```python
from build123d import *

# Parameters (mm, degrees)
BOSS_EXTRUDE1_DEPTH = 1.8
SKETCH2_R           = 2.500000000000001
BOSS_EXTRUDE2_DEPTH = 3
SKETCH3_R           = 2.5000000000000013
BOSS_EXTRUDE3_DEPTH = 0.5
CHAMFER1_SIZE       = 0.4
SKETCH4_W           = 0.5
SKETCH4_H           = 1.7000000000000002
BOSS_EXTRUDE4_DEPTH = 0.2
CHAMFER2_SIZE       = 0.3
CHAMFER2_SIZE_2     = 0.221880218
FILLET1_R           = 0.2


with BuildPart() as part:
    # Sketch1 → Boss-Extrude1 (new body)
    with BuildSketch(Plane(origin=(0, 0, 0), x_dir=(1, 0, 0), z_dir=(0, 1, 0))):
        with BuildLine():
            Line((-3, -6.5), (-3.0000000000000027, 6.499999999999998))
            ThreePointArc((-3.0000000000000027, 6.499999999999998), (-4.2e-15, 9.5), (2.9999999999999973, 6.500000000000002))
            Line((2.9999999999999973, 6.500000000000002), (3, -6.5))
            ThreePointArc((3, -6.5), (-5.5e-16, -9.5), (-3, -6.5))
        make_face()
    extrude(amount=BOSS_EXTRUDE1_DEPTH)

    # Sketch2 → Boss-Extrude2 (add)
    with BuildSketch(Plane(origin=(0, 1.8, 0), x_dir=(1, 0, 0), z_dir=(0, 1, 0))):
        with Locations(Location((-2.39e-15, 6.5, 0), (0, 0, 270))):
            Circle(SKETCH2_R)
        with Locations(Location((0, -6.5, 0), (0, 0, 270))):
            Circle(SKETCH2_R)
    extrude(amount=BOSS_EXTRUDE2_DEPTH)

    # Sketch3 → Boss-Extrude3 (add)
    with BuildSketch(Plane(origin=(0, 4.800000000000001, 0), x_dir=(1, 0, 0), z_dir=(0, 1, 0))):
        with Locations(Location((-2.39e-15, 6.5, 0), (0, 0, 270))):
            Circle(SKETCH3_R)
    extrude(amount=BOSS_EXTRUDE3_DEPTH)

    # Chamfer1
    chamfer1_edges = [part.edges().sort_by_distance(p)[0] for p in [
        (7.7e-16, 4.8, 3.999999999999999),
        (-1.62e-15, 5.300000000000001, -9.000000000000002),
    ]]
    chamfer(chamfer1_edges, length=CHAMFER1_SIZE)

    # Sketch4 → Boss-Extrude4 (add)
    with BuildSketch(Plane(origin=(0, 5.300000000000001, 0), x_dir=(1, 0, 0), z_dir=(0, 1, 0))):
        with BuildLine():
            Line((-0.75, 7.913329402510258), (-0.75, 7.304673846971556))
            ThreePointArc((-0.75, 7.304673846971556), (-4.54e-15, 5.4), (0.75, 7.304673846971556))
            Line((0.75, 7.304673846971556), (0.75, 7.913329402510258))
            ThreePointArc((0.75, 7.913329402510258), (-5.52e-15, 4.9), (-0.75, 7.913329402510258))
        make_face()
        with Locations((-2.76e-15, 7.449999999999999)):
            Rectangle(SKETCH4_W, SKETCH4_H)
    extrude(amount=BOSS_EXTRUDE4_DEPTH)

    # Chamfer2
    # the kernel refuses this chamfer: 0.3, 0.221880218 mm, written as the material it takes off along each edge
    with BuildSketch(Plane(origin=(-0.75, 5.300000000000001, -7.913329402510258), x_dir=(0, 0, 1), z_dir=(0, 1, 0))) as chamfer2_piece_1:
        with BuildLine():
            Line((CHAMFER2_SIZE, 0), (0.11497408326020686, -0.18502591673979885))
            ThreePointArc((0.11497408326020686, -0.18502591673979885), (0.05505412011014688, -0.09562891224277614), (0, 0))
            Line((0, 0), (CHAMFER2_SIZE, 0))
        make_face()
    extrude(amount=0.9715048963897726, mode=Mode.SUBTRACT)
    with BuildSketch(Plane(origin=(0.75, 5.300000000000001, -7.913329402510258), x_dir=(0.8394299671515956, 0, 0.5434678741635711), z_dir=(0, 1, 0))) as chamfer2_piece_2:
        with BuildLine():
            Line((0.27705330102285075, 2e-17), (CHAMFER2_SIZE_2 * 0.543467874804, -CHAMFER2_SIZE_2 * 0.83942996814))
            Line((CHAMFER2_SIZE_2 * 0.543467874804, -CHAMFER2_SIZE_2 * 0.83942996814), (0, 0))
            ThreePointArc((0, 0), (0.14238943823073183, 0.00600337759415658), (0.27705330102285075, 2e-17))
        make_face()
    extrude(amount=0.9123006442989672, mode=Mode.SUBTRACT)

    # Fillet1
    # the kernel refuses this fillet: 0.2 mm, written as the material it takes off along each edge
    with BuildSketch(Plane(origin=(-0.7500000000000032, 5.500000000000001, -6.599999999999999), x_dir=(0, -1, 0), z_dir=(1, 0, 0))) as fillet1_piece_1:
        with BuildLine():
            CenterArc((FILLET1_R, FILLET1_R), FILLET1_R, 180, 90)
            Line((0, FILLET1_R), (0, 0))
            Line((0, 0), (FILLET1_R, 0))
        make_face()
    extrude(amount=1.5000000000000009, mode=Mode.SUBTRACT)
    with BuildSketch(Plane(origin=(-0.2500000000000028, 5.500000000000001, -8.799999999999999), x_dir=(0, -1, 0), z_dir=(0, 0, 1)), Plane(origin=(0.24999999999999725, 5.500000000000001, -6.099999999999998), x_dir=(0, -1, 0), z_dir=(0, 0, -1))) as fillet1_piece_2:
        with BuildLine():
            CenterArc((FILLET1_R, FILLET1_R), FILLET1_R, 180, 90)
            Line((0, FILLET1_R), (0, 0))
            Line((0, 0), (FILLET1_R, 0))
        make_face()
    extrude(amount=2.700000000000001, mode=Mode.SUBTRACT)
    with BuildSketch(Plane(origin=(0.7499999999999977, 5.500000000000001, -8.299999999999999), x_dir=(0, -1, 0), z_dir=(-1, 0, 0))) as fillet1_piece_3:
        with BuildLine():
            CenterArc((FILLET1_R, FILLET1_R), FILLET1_R, 180, 90)
            Line((0, FILLET1_R), (0, 0))
            Line((0, 0), (FILLET1_R, 0))
        make_face()
    extrude(amount=1.5000000000000009, mode=Mode.SUBTRACT)
    with BuildSketch(Plane(origin=(-0.75, 5.500000000000001, -8.11332940251), x_dir=(0, -1, 0), z_dir=(0, 0, 1))) as fillet1_piece_4:
        with BuildLine():
            CenterArc((FILLET1_R, -FILLET1_R), FILLET1_R, 90, 90)
            Line((0, -FILLET1_R), (0, 0))
            Line((0, 0), (FILLET1_R, 0))
        make_face()
    extrude(amount=1.3086555555384454, mode=Mode.SUBTRACT)
    with BuildSketch(Plane(origin=(-8e-17, 5.500000000000001, -6.500000000000001), x_dir=(-0.2897858618854929, 0, -0.9570915077730457), z_dir=(0.9570915077730457, 0, -0.2897858618854929))) as fillet1_piece_5:
        with BuildLine():
            CenterArc((1.1000000000000005 + FILLET1_R, -FILLET1_R), FILLET1_R, 90.00000000000006, 89.99999999999994)
            Line((1.1000000000000005 + FILLET1_R, 0), (1.1000000000000005, 0))
            Line((1.1000000000000005, 0), (1.1000000000000005, -FILLET1_R))
        make_face()
    revolve(axis=Axis((-8e-17, 5.500000000000001, -6.500000000000001), (0, 1, 0)), revolution_arc=326.3097273547943, mode=Mode.SUBTRACT)
    with BuildSketch(Plane(origin=(0.75, 5.500000000000001, -6.804673846971555), x_dir=(0, -1, 0), z_dir=(0, 0, -1))) as fillet1_piece_6:
        with BuildLine():
            CenterArc((FILLET1_R, -FILLET1_R), FILLET1_R, 90, 90)
            Line((0, -FILLET1_R), (0, 0))
            Line((0, 0), (FILLET1_R, 0))
        make_face()
    extrude(amount=1.3867753372771254, mode=Mode.SUBTRACT)
    with BuildSketch(Plane(origin=(8e-17, 5.500000000000001, -6.500000000000001), x_dir=(0.3405261643731297, 0, -0.9402350404964305), z_dir=(-0.9402350404964305, 0, -0.3405261643731297))) as fillet1_piece_7:
        with BuildLine():
            CenterArc((1.5999999999999999 - FILLET1_R, FILLET1_R), FILLET1_R, 270, 90)
            Line((1.5999999999999999 - FILLET1_R, 0), (1.5999999999999999, 0))
            Line((1.5999999999999999, 0), (1.5999999999999999, FILLET1_R))
        make_face()
    revolve(axis=Axis((8e-17, 5.500000000000001, -6.500000000000001), (0, -1, 0)), revolution_arc=322.309003529889, mode=Mode.SUBTRACT)


solid = part.part
```
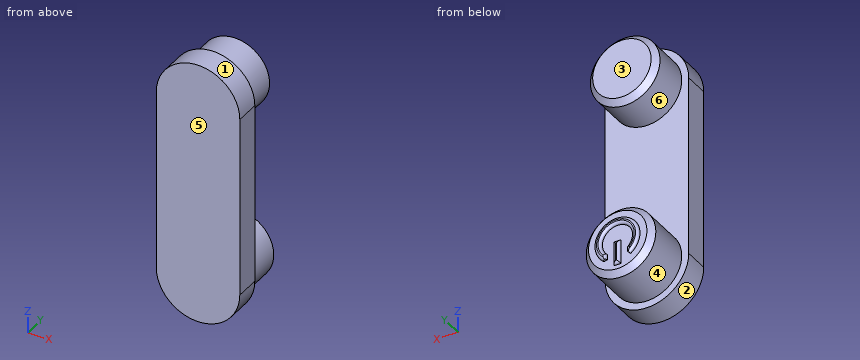
CAD build for the part. Positions are in the model's coordinates, mm. Face numbers are marked on the shaded views. A direction names the side the tool comes from. Round coordinates to 2 decimals unless told otherwise and drop trailing zeros. Write each loop counter-clockwise with the first axis right and the second up, starting at its lowest first coordinate (ties: lowest second). Pieces come first, ordered by that corner, then holes. Notation, with made-up numbers: M 12.25,-20.5 L 60.25,-20.5 A15 cw 60.25,-8.5 Z; hole C 51.25,-3.75 d9. An arc over 180 degrees is marked long. One line per question, with ' | ' between items.
1. Cut at B-B on y = 0.45. Write the cut outline in (x, z).
Working result:
outline: M -3,-6.5 A3 ccw 3,-6.5 L 3,6.5 A3 ccw -3,6.5 Z
2. Mould opens along Z. For the marked faces 1, 2, 3 and 4 say: pulls with the +Z half, pulls with the -Z half, needs draft (parallel to the pull), parting line crosses it, or undercut.
Working result:
face 1: pulls with the +Z half | face 2: pulls with the -Z half | face 3: needs draft | face 4: undercut
3. Which spindle directions (+Z, -Z, +X, -X, +Y, -Y) get a long thin tool onto all of the face, cutting with end or side? Do the marked faces 5 and 6. Say none if no direction does.
Working result:
face 5: +Z, -Z, +X, -X, -Y | face 6: +Y
4. Cut at A-A on z = 1.25. Write the cut outline in (x, y), and give its area (3 significant figures).
Working result:
outline: M -3,0 L 3,0 L 3,1.8 L -3,1.8 Z | area: 10.8 mm2
5. Pin check, flat tips, straight feed: pin 1 Ø3 at (x, y) = (-0.5, 3.5) entering from +Z; pin 2 Ø1.3 at (x, z) = (0.5, 7.5) entering from +Y. Stop position of each tip, or through.
Working result:
pin 1: z = 9 | pin 2: y = 4.8
6. Probe L1, parallel to Y at x = 2.5, z = -1.5; L2, parallel to Y at x = 1.5, z = 6.5; L3, parallel to Z at x = 2.25, y = 3.4. List the from-to ranges inside material, lowest first. Write a range as from..to.
Working result:
L1: 0..1.8 | L2: 0..4.8 | L3: -7.59..-5.41, 5.41..7.59
